Can you work these out from the model? Positions are in its coordinate system, mm. Face numbers are marked on the shaded views. A direction names the side the tool comes from. Round coordinates to 2 decimals unless told otherwise and drop trailing zeros. Loops run counter-clockwise (first coordinate to the right, second up) from the corner with the lowest first, then second, coordinate; pieces in that order, holes last. Notation, with made-up numbers: M -16,-14 L 25,-14 A37 cw 25,24 Z; hole C 51.25,89.25 d1. An arc over 180 degrees is marked long. Use a Markdown table: item, result. Add a question column.
```python
from build123d import *

# Parameters (mm, degrees)
SKETCH1_R               = 7.18463753
BOSS_EXTRUDE1_DEPTH     = 4.5
CUT_EXTRUDE2_START      = 4
SKETCH4_R               = 2
CUT_EXTRUDE2_DEPTH      = 29
SKETCH4_4_R             = 2
CUT_EXTRUDE3_DEPTH      = 29
CUT_EXTRUDE4_DEPTH      = 29
CUT_EXTRUDE4_DEPTH_BACK = 29


with BuildPart() as part:
    # Sketch1 → Boss-Extrude1 (new body, symmetric)
    with BuildSketch(Plane.XY):
        with BuildLine():
            Line((-1.254341559, 11.934262744), (-28.289662127, 9.092736051))
            ThreePointArc((-28.289662127, 9.092736051), (-43.850490966, 9.48747573), (-58.786122703, 13.871779345))
            ThreePointArc((-58.786122703, 13.871779345), (-74.520010862, 15.355444557), (-88, 7.106420865))
            Line((-88, 7.106420865), (-86.5, 4.508344654))
            Line((-86.5, 4.508344654), (-81.303847577, 7.508344654))
            Line((-81.303847577, 7.508344654), (-76.107695155, 4.508344654))
            Line((-76.107695155, 4.508344654), (-66.705771366, -11.776265037))
            ThreePointArc((-66.705771366, -11.776265037), (-56.482680545, -7.851988144), (-45.547275152, -7.278887832))
            Line((-45.547275152, -7.278887832), (-1.254341559, -11.934262744))
            ThreePointArc((-1.254341559, -11.934262744), (12, 0), (-1.254341559, 11.934262744))
        make_face()
        Circle(SKETCH1_R, mode=Mode.SUBTRACT)
        with BuildLine():
            Line((-69.509618943, 5.080141424), (-63.509618943, -5.312163422))
            Line((-63.509618943, -5.312163422), (-57.447441117, -1.812163422))
            ThreePointArc((-57.447441117, -1.812163422), (-56.98151529, -1.204957063), (-57.081415713, -0.446138018))
            Line((-57.081415713, -0.446138018), (-62.081415713, 8.21411602))
            ThreePointArc((-62.081415713, 8.21411602), (-62.688622072, 8.680041846), (-63.447441117, 8.580141424))
            Line((-63.447441117, 8.580141424), (-69.509618943, 5.080141424))
        make_face(mode=Mode.SUBTRACT)
    extrude(amount=BOSS_EXTRUDE1_DEPTH, both=True)

    # Sketch4 → Cut-Extrude2 (cut)
    with BuildSketch(Plane(origin=(-23.5771705, 40.836857204, 0), x_dir=(0.866025404, 0.5, 0), z_dir=(0.5, -0.866025404, 0)).offset(CUT_EXTRUDE2_START)):
        with Locations((-53.6570251, 0)):
            Circle(SKETCH4_R)
    extrude(amount=CUT_EXTRUDE2_DEPTH, mode=Mode.SUBTRACT)

    # Sketch4_4 → Cut-Extrude3 (cut)
    with BuildSketch(Plane(origin=(-23.5771705, 40.836857204, 0), x_dir=(0.866025404, 0.5, 0), z_dir=(0.5, -0.866025404, 0))):
        with BuildLine():
            Line((-66.6570251, -1.25), (-62.2182746, -1.25))
            ThreePointArc((-62.2182746, -1.25), (-62.6570251, 0), (-62.2182746, 1.25))
            Line((-62.2182746, 1.25), (-66.6570251, 1.25))
            Line((-66.6570251, 1.25), (-66.6570251, -1.25))
        make_face()
        with Locations((-60.6570251, 0)):
            Circle(SKETCH4_4_R)
        with BuildLine():
            Line((-59.095775601, -1.25), (-57.6570251, -1.25))
            Line((-57.6570251, -1.25), (-57.6570251, 1.25))
            Line((-57.6570251, 1.25), (-59.095775601, 1.25))
            ThreePointArc((-59.095775601, 1.25), (-58.769897786, 0.662382443), (-58.6570251, 0))
            ThreePointArc((-58.6570251, 0), (-58.769897786, -0.662382443), (-59.095775601, -1.25))
        make_face()
    extrude(amount=CUT_EXTRUDE3_DEPTH, mode=Mode.SUBTRACT)

    # Sketch4_6 → Cut-Extrude4 (cut, two sides)
    with BuildSketch(Plane(origin=(-23.5771705, 40.836857204, 0), x_dir=(0.866025404, 0.5, 0), z_dir=(0.5, -0.866025404, 0))) as cut_extrude4_sk:
        Polygon((-72.6570251, 2), (-56.790792146, 4.5), (-72.6570251, 4.5), align=None)
        Polygon((-56.790792146, -4.5), (-72.6570251, -4.5), (-72.6570251, -2), align=None)
    extrude(amount=CUT_EXTRUDE4_DEPTH, mode=Mode.SUBTRACT)
    extrude(cut_extrude4_sk.sketch, amount=-CUT_EXTRUDE4_DEPTH_BACK, mode=Mode.SUBTRACT)


solid = part.part
```
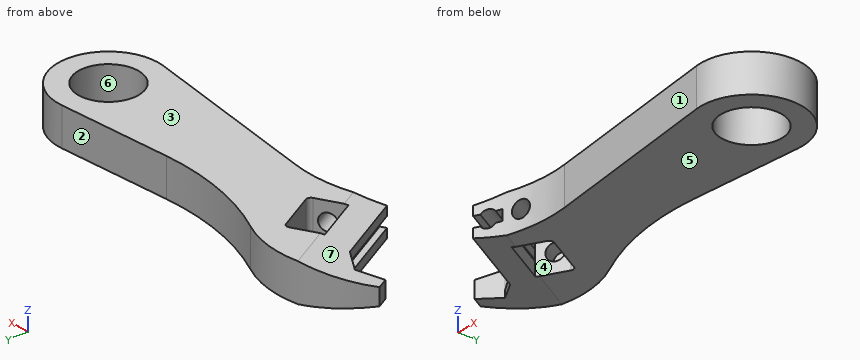
(1) On a 3-axis mill with a long thin cutter (end or side, diameter ignored), from which of +Z, -Z, +X, -X, +Y, -Y can I reach the whole of each face in a straight line? I mean the marked faces 1, 2 and 3. Say none if no direction works.
(2) I'm going to push flat-ended pins straight in: pin 1 (11.5 mm diameter, centred on x = 0, y = 0, fed in from -Z); pin 2 (1 mm diameter, centred on x = -63.5, z = 0, fed in from -Y); pin 3 (1.5 mm diameter, centred on x = -22.5, z = -1.5, fed in from -Y); pin 4 (12.5 mm diameter, centred on x = -70.5, y = -4.5, fed in from -Z). Where does each tip first touch, or does it pass through?
(3) Thinking about a two-plate mould opening in Y: for the marked faces 4, 5, 6 and 7, which applies, released by +Y, released by -Y, zero draft, split by the parting line, or undercut?
(4) Suppose I cut it at A-A on x = 4.5. List the corners of the cut face in (y, z) for me.
(5) If I drill on probe 1 along Y at (x, z) = (0, 1.5); probe 2 along X at (y, z) = (4.75, -3); probe 3 along X at (y, z) = (-4.25, 2.75), over which ranges is the centre line in solid material (lowest first)? Write a range as [from, to].
Results below:
| question | item | result |
|---|---|---|
| 1 | face 1 | +Z, -Z, -Y |
| 1 | face 2 | +Z, -Z, +Y |
| 1 | face 3 | +Z, +X, -X, +Y, -Y |
| 2 | pin 1 | passes through |
| 2 | pin 2 | stops at y = -6.19 |
| 2 | pin 3 | stops at y = -9.78 |
| 2 | pin 4 | stops at z = -4.36 |
| 3 | face 4 | undercut |
| 3 | face 5 | zero draft |
| 3 | face 6 | undercut |
| 3 | face 7 | released by -Y |
| 4 | outline | M -11.12,-4.5 L -5.6,-4.5 L -5.6,4.5 L -11.12,4.5 Z; M 5.6,-4.5 L 11.12,-4.5 L 11.12,4.5 L 5.6,4.5 Z |
| 5 | probe 1 | y = [-12, -7.18], [7.18, 12] |
| 5 | probe 2 | x = [-76.53, -69.32], [-60.08, -5.39], [5.39, 11.02] |
| 5 | probe 3 | x = [-71.05, -64.12], [-61.67, -5.79], [5.79, 11.22] |
